```python
from build123d import *

# Parameters (mm, degrees)
SKETCH1_R           = 20
BOSS_EXTRUDE1_DEPTH = 30
SKETCH2_R           = 50
BOSS_EXTRUDE2_DEPTH = 30
CHAMFER1_SIZE       = 7.5
CUT_EXTRUDE1_DEPTH  = 5


with BuildPart() as part:
    # Sketch1 → Boss-Extrude1 (new body)
    with BuildSketch(Plane(origin=(0, 0, 0), x_dir=(1, 0, 0), z_dir=(0, 1, 0))):
        Circle(SKETCH1_R)
    extrude(amount=BOSS_EXTRUDE1_DEPTH)

    # Sketch2 → Boss-Extrude2 (add)
    with BuildSketch(Plane(origin=(0, 30, 0), x_dir=(1, 0, 0), z_dir=(0, 1, 0))):
        Circle(SKETCH2_R)
    extrude(amount=BOSS_EXTRUDE2_DEPTH)

    # Chamfer1
    chamfer1_edges = [part.edges().sort_by_distance(p)[0] for p in [
        (-50, 60, 0),
    ]]
    chamfer(chamfer1_edges, length=CHAMFER1_SIZE)

    # Sketch3 → Cut-Extrude1 (cut)
    with BuildSketch(Plane(origin=(0, 60, 0), x_dir=(1, 0, 0), z_dir=(0, 1, 0))):
        with BuildLine():
            Line((47.051270189, -18.504809472), (7.5, 4.330127019))
            Line((7.5, 4.330127019), (7.5, 50))
            ThreePointArc((7.5, 50), (0, 57.5), (-7.5, 50))
            Line((-7.5, 50), (-7.5, 4.330127019))
            Line((-7.5, 4.330127019), (-47.051270189, -18.504809472))
            ThreePointArc((-47.051270189, -18.504809472), (-49.796460718, -28.75), (-39.551270189, -31.495190528))
            Line((-39.551270189, -31.495190528), (0, -8.660254038))
            Line((0, -8.660254038), (39.551270189, -31.495190528))
            ThreePointArc((39.551270189, -31.495190528), (49.796460718, -28.75), (47.051270189, -18.504809472))
        make_face()
    extrude(amount=-CUT_EXTRUDE1_DEPTH, mode=Mode.SUBTRACT)


solid = part.part
```
Part model, mm, in its own coordinate system. A direction names the side the tool comes from. Round coordinates to 2 decimals unless told otherwise and drop trailing zeros. Loops run counter-clockwise (first coordinate to the right, second up) from the corner with the lowest first, then second, coordinate; pieces in that order, holes last.
1. Drill centre lines: line 1 along Y through (x, z) = (-12, -24); line 2 along Y through (x, z) = (-14, 15); line 3 along X through (y, z) = (12.5, -3). Where is each one in solid material? Low to high.
Solutions:
line 1: y = 30 to 60
line 2: y = 30 to 55
line 3: x = -19.77 to 19.77
2. Slice it at A-A (z = 0). Give the cut face in (x, y), and give its area (3 significant figures).
Solutions:
outline: (-50, 30) - (-20, 30) - (-20, 0) - (20, 0) - (20, 30) - (50, 30) - (50, 52.5) - (42.5, 60) - (15, 60) - (15, 55) - (-15, 55) - (-15, 60) - (-42.5, 60) - (-50, 52.5) - close
area: 3,990 mm2
3. Flat gauge pins, fed straight in: pin 1 (12 mm diameter, centred on y = 21.5, z = 29.5, fed in from +X); pin 2 (8 mm diameter, centred on x = -7, y = 11.5, fed in from -Z); pin 3 (4 mm diameter, centred on y = 36, z = 7.5, fed in from -X); pin 4 (2.5 mm diameter, centred on y = 58, z = -27.5, fed in from +X). Where does each tip first touch, or does it go through?
Solutions:
pin 1: passes through
pin 2: stops at z = -19.77
pin 3: stops at x = -49.7
pin 4: stops at x = 36.82
4. Two-plate mould, pull along X, no slides. Class faces 5 (the face through (0, 0, 0)), 6 (the face through (26.19, 57.54, 6.46)), 7 (the face through (47.69, 41.09, -15.02)): pulls with the +X half, pulls with the -X half, needs draft (parallel to the pull), parting line crosses it, or undercut.
Solutions:
face 5: needs draft
face 6: undercut
face 7: parting line crosses it
5. 3-axis set-ups, long thin cutter, end or side, ignore diameter. For faces 1 (the face through (7.5, 58, -25)), 2 (the face through (-25.677, 57.535, 6.164)), 3 (the face through (25, 60, -14)), 4 (the face through (-4.336, 14.79, 19.524)): which of +Z, -Z, +X, -X, +Y, -Y reach the whole face in a straight line?
Solutions:
face 1: -Z, +Y
face 2: +Y
face 3: +Z, -Z, +X, -X, +Y
face 4: -Y
6. Slice it at B-B (y = 26). Give the cut face in (x, z).
Solutions:
outline: circle Ø40 at (0, 0)
